from build123d import *

# Parameters (mm, degrees)
SKETCH1_W           = 1.5
SKETCH1_H           = 40
BOSS_EXTRUDE1_DEPTH = 40
SKETCH2_W           = 40
SKETCH2_H           = 1.5
BOSS_EXTRUDE2_DEPTH = 20.5
SKETCH3_R           = 1.5
CUT_EXTRUDE1_DEPTH  = 20.5
FILLET5_R           = 1.5
FILLET6_R           = 1.5
FILLET7_R           = 10
FILLET8_R           = 10
FILLET9_R           = 1.5
FILLET10_R          = 1.5
SKETCH6_R           = 1.5
CUT_EXTRUDE2_DEPTH  = 4
SKETCH7_R           = 12.9
CUT_EXTRUDE5_DEPTH  = 4


with BuildPart() as part:
    # Sketch1 → Boss-Extrude1 (new body)
    with BuildSketch(Plane(origin=(0, 0, 0), x_dir=(1, 0, 0), z_dir=(0, 1, 0))):
        with Locations((0.75, -20)):
            Rectangle(SKETCH1_W, SKETCH1_H)
    extrude(amount=BOSS_EXTRUDE1_DEPTH)

    # Sketch2 → Boss-Extrude2 (add)
    with BuildSketch(Plane(origin=(1.5, 0, 0), x_dir=(0, 0, -1), z_dir=(1, 0, 0))):
        with Locations((-20, 0.75)):
            Rectangle(SKETCH2_W, SKETCH2_H)
    extrude(amount=BOSS_EXTRUDE2_DEPTH)

    # Sketch3 → Cut-Extrude1 (cut)
    with BuildSketch(Plane(origin=(0, 1.5, 0), x_dir=(1, 0, 0), z_dir=(0, 1, 0))):
        with Locations(Location((6, -5, 0), (0, 0, 270))):
            Circle(SKETCH3_R)
        with Locations(Location((6, -35, 0), (0, 0, 270))):
            Circle(SKETCH3_R)
        with Locations(Location((12, -35, 0), (0, 0, 270))):
            Circle(SKETCH3_R)
        with Locations(Location((12, -5, 0), (0, 0, 270))):
            Circle(SKETCH3_R)
        with Locations(Location((18, -5, 0), (0, 0, 270))):
            Circle(SKETCH3_R)
        with Locations(Location((18, -35, 0), (0, 0, 270))):
            Circle(SKETCH3_R)
    extrude(amount=-CUT_EXTRUDE1_DEPTH, mode=Mode.SUBTRACT)

    # Fillet5
    fillet5_edges = [part.edges().sort_by_distance(p)[0] for p in [
        (0, 0, 20),
    ]]
    fillet(fillet5_edges, radius=FILLET5_R)

    # Fillet6
    fillet6_edges = [part.edges().sort_by_distance(p)[0] for p in [
        (1.5, 1.5, 20),
    ]]
    fillet(fillet6_edges, radius=FILLET6_R)

    # Fillet7
    fillet7_edges = [part.edges().sort_by_distance(p)[0] for p in [
        (0.75, 40, 40),
    ]]
    fillet(fillet7_edges, radius=FILLET7_R)

    # Fillet8
    fillet8_edges = [part.edges().sort_by_distance(p)[0] for p in [
        (0.75, 40, 0),
    ]]
    fillet(fillet8_edges, radius=FILLET8_R)

    # Fillet9
    fillet9_edges = [part.edges().sort_by_distance(p)[0] for p in [
        (22, 0.75, 40),
    ]]
    fillet(fillet9_edges, radius=FILLET9_R)

    # Fillet10
    fillet10_edges = [part.edges().sort_by_distance(p)[0] for p in [
        (22, 0.75, 0),
    ]]
    fillet(fillet10_edges, radius=FILLET10_R)

    # Sketch6 → Cut-Extrude2 (cut)
    with BuildSketch(Plane(origin=(1.5, 0, 0), x_dir=(0, 0, -1), z_dir=(1, 0, 0))):
        with Locations((-20, 36.5)):
            Circle(SKETCH6_R)
        with Locations((-12.75, 34.557368355)):
            Circle(SKETCH6_R)
        with Locations((-7.442631645, 29.25)):
            Circle(SKETCH6_R)
        with Locations((-5.5, 22)):
            Circle(SKETCH6_R)
        with Locations((-7.442631645, 14.75)):
            Circle(SKETCH6_R)
        with Locations((-12.75, 9.442631645)):
            Circle(SKETCH6_R)
        with Locations((-20, 7.5)):
            Circle(SKETCH6_R)
        with Locations((-27.25, 9.442631645)):
            Circle(SKETCH6_R)
        with Locations((-32.557368355, 14.75)):
            Circle(SKETCH6_R)
        with Locations((-34.5, 22)):
            Circle(SKETCH6_R)
        with Locations((-32.557368355, 29.25)):
            Circle(SKETCH6_R)
        with Locations((-27.25, 34.557368355)):
            Circle(SKETCH6_R)
    extrude(amount=-CUT_EXTRUDE2_DEPTH, mode=Mode.SUBTRACT)

    # Sketch7 → Cut-Extrude5 (cut)
    with BuildSketch(Plane.ZY):
        with Locations((20, 22)):
            Circle(SKETCH7_R)
    extrude(amount=-CUT_EXTRUDE5_DEPTH, mode=Mode.SUBTRACT)


solid = part.part
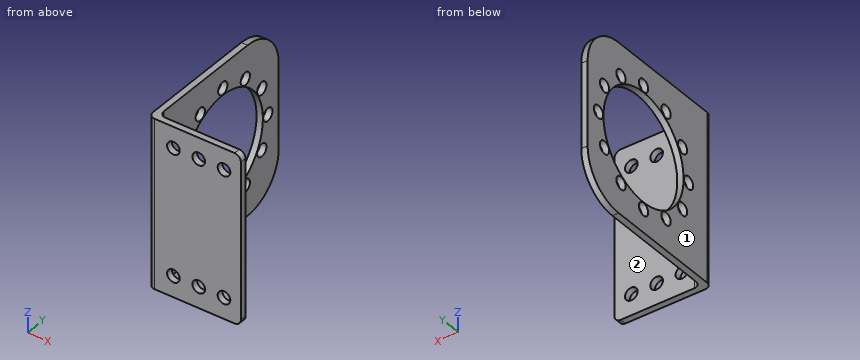
Source: CAD feature listing. Evaluate the final solid. Frame: model axes, mm. Face numbers are marked on the shaded views. A direction names the side the tool comes from. Round coordinates to 2 decimals unless told otherwise and drop trailing zeros. Write each loop counter-clockwise with the first axis right and the second up, starting at its lowest first coordinate (ties: lowest second). Pieces come first, ordered by that corner, then holes. Notation, with made-up numbers: M 11,4 L 68,4 A15 cw 68,26 Z; hole C 81.25,67.25 d4. An arc over 180 degrees is marked long. One line per item, written item: value. Start each with the question number.
Item 1: Ray query, L1, parallel to X at y = 1, z = 35; L2, parallel to Y at x = 13.25, z = 10; L3, parallel to X at y = 0.75, z = 35. Return the intervals inside material, ascending. Write a range as from..to.
Item 2: Section query A-A (y = 22). Return the cut outline in (x, z), plus the area to 3 significant figures.
Item 3: Pin query (flat end, axial travel): pin 1 (2.5 mm diameter, centred on y = 14.75, z = 32.56, fed in from +X); pin 2 (4 mm diameter, centred on y = 14.75, z = 7.44, fed in from +X); pin 3 (10 mm diameter, centred on x = 14.5, z = 16, fed in from +Y). Return the tip coordinate at first contact, or that it passes through.
Item 4: Section query C-C (x = 18). Return the cut outline in (y, z), plus the area to 3 significant figures.
Item 5: Section query B-B (z = 20). Return the cut outline in (x, y), plus the area to 4 significant figures.
Item 6: Set-up query: the marked faces 1 and 2. Return all of +Z, -Z, +X, -X, +Y, -Y with unobstructed straight access to the full face (end or side cutting, diameter ignored); none if empty.
Item 7: Section query D-D (y = 7). Return the cut outline in (x, z), plus the area to 3 significant figures.
Result set:
1. L1: x = 0.09..4.5, 7.5..10.5, 13.5..16.5, 19.5..22
1. L2: y = 0..1.5
1. L3: x = 0.2..4.5, 7.5..10.5, 13.5..16.5, 19.5..22
2. outline: M 0,0 L 1.5,0 L 1.5,4 L 0,4 Z; M 0,7 L 1.5,7 L 1.5,7.1 L 0,7.1 Z; M 0,32.9 L 1.5,32.9 L 1.5,33 L 0,33 Z; M 0,36 L 1.5,36 L 1.5,40 L 0,40 Z
2. area: 12.3 mm²
3. pin 1: passes through
3. pin 2: stops at x = 1.5
3. pin 3: stops at y = 1.5
4. outline: M 0,0 L 1.5,0 L 1.5,3.5 L 0,3.5 Z; M 0,6.5 L 1.5,6.5 L 1.5,33.5 L 0,33.5 Z; M 0,36.5 L 1.5,36.5 L 1.5,40 L 0,40 Z
4. area: 51.0 mm²
5. outline: M 0,1.5 A1.5 ccw 1.5,0 L 22,0 L 22,1.5 L 3,1.5 A1.5 cw 1.5,3 L 1.5,6 L 0,6 Z; M 0,9 L 1.5,9 L 1.5,9.1 L 0,9.1 Z; M 0,34.9 L 1.5,34.9 L 1.5,35 L 0,35 Z; M 0,38 L 1.5,38 L 1.5,40 L 0,40 Z
5. area: 43.05 mm²
6. face 1: +Z, -Z, -X, +Y, -Y
6. face 2: +Z, -Z, +X, +Y
7. outline: M 0,0 L 1.5,0 L 1.5,18.59 L 0,18.59 Z; M 0,21.41 L 1.5,21.41 L 1.5,40 L 0,40 Z
7. area: 55.8 mm²
